Can you work these out from the drawing? Everything is in mm from the part's minimum corner. A direction names the side the tool comes from. Round coordinates to 2 decimals unless told otherwise and drop trailing zeros. Write each loop counter-clockwise with the first axis right and the second up, starting at its lowest first coordinate (ties: lowest second). Pieces come first, ordered by that corner, then holes. Notation, with made-up numbers: M 30,73 L 58,73 A23 cw 58,101 Z; hole C 26,73 d5. An arc over 180 degrees is marked long. Use a Markdown table: item, result. Add a question column.
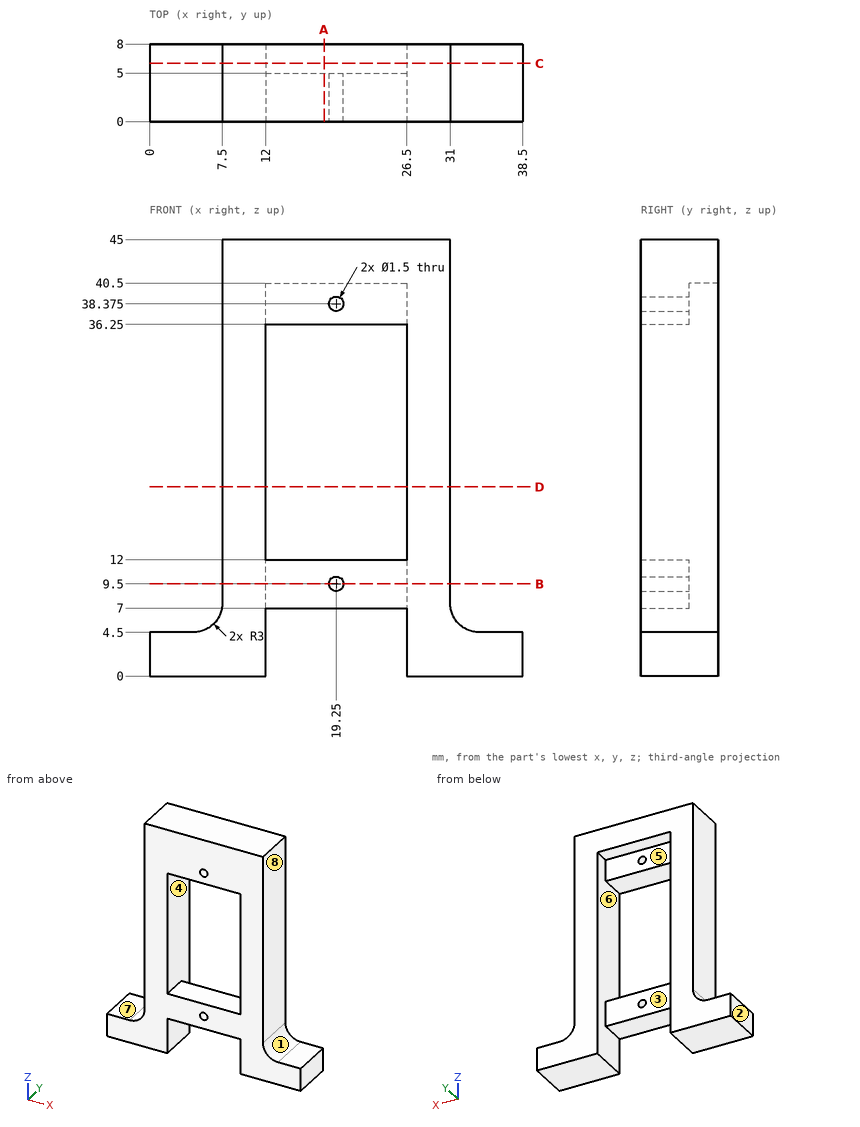
Item 1: Imagine slicing it at C-C on y = 6. List the corners of the cut face in (x, z) for me, plus the area to 3 significant figures.
Item 2: I need wall thicknesses on probe 1 along Z at (x, y) = (19.25, 1.4) (3 decimals); probe 2 along Z at (x, y) = (23.5, 4.5); probe 3 along X at (y, z) = (0.75, 17). Which ranges of each line are inside material? Lowest first, please. Write a range as from..to.
Item 3: Imagine slicing it at A-A on x = 18. List the corners of the cut face in (y, z) for me.
Item 4: For pin 1 Ø3.5 at (x, y) = (1.5, 4.5) entering from +Z; pin 2 Ø1.7 at (x, z) = (19.25, 38.375) entering from +Y; pin 3 Ø0.9 at (x, z) = (19.25, 9.5) entering from +Y; pin 4 Ø2.5 at (x, y) = (17, 6.5) entering from -Z, each with a flat end and sliding along its axis, tell me the tip position at first contact or that it passes through.
Item 5: Imagine slicing it at D-D on z = 19.5. List the corners of the cut face in (x, y) for me.
Item 6: If we mould it in two halves opening along X, with no side actions, what happens to the marked faces 1, 2, 3 and 4? For each: +X half, -X half, draft (parallel to the pull), parting line (faces both ways), or undercut.
Item 7: On a 3-axis mill with a long thin cutter (end or side, diameter ignored), from which of +Z, -Z, +X, -X, +Y, -Y can I reach the whole of each face in a straight line? I mean the marked faces 5, 6, 7 and 8. Say none if no direction works.
Item 8: Imagine slicing it at B-B on z = 9.5. List the corners of the cut face in (x, y) for me.
The answers:
| question | item | result |
|---|---|---|
| 1 | outline | M 0,0 L 12,0 L 12,40.5 L 26.5,40.5 L 26.5,0 L 38.5,0 L 38.5,4.5 L 34,4.5 A3 cw 31,7.5 L 31,45 L 7.5,45 L 7.5,7.5 A3 cw 4.5,4.5 L 0,4.5 Z |
| 1 | area | 542 mm² |
| 2 | probe 1 | 7..8.75, 10.25..12, 36.25..37.625, 39.125..45 |
| 2 | probe 2 | 7..12, 36.25..45 |
| 2 | probe 3 | 7.5..12, 26.5..31 |
| 3 | outline | M 0,7 L 5,7 L 5,12 L 0,12 Z; M 0,36.25 L 5,36.25 L 5,40.5 L 8,40.5 L 8,45 L 0,45 Z |
| 4 | pin 1 | z = 4.5 |
| 4 | pin 2 | y = 5 |
| 4 | pin 3 | through |
| 4 | pin 4 | z = 40.5 |
| 5 | outline | M 7.5,0 L 12,0 L 12,8 L 7.5,8 Z; M 26.5,0 L 31,0 L 31,8 L 26.5,8 Z |
| 6 | face 1 | +X half |
| 6 | face 2 | -X half |
| 6 | face 3 | undercut |
| 6 | face 4 | undercut |
| 7 | face 5 | -Z, +Y |
| 7 | face 6 | +Y |
| 7 | face 7 | +Z, -X, +Y, -Y |
| 7 | face 8 | +Z, +X, +Y, -Y |
| 8 | outline | M 7.5,0 L 18.5,0 L 18.5,5 L 12,5 L 12,8 L 7.5,8 Z; M 20,0 L 31,0 L 31,8 L 26.5,8 L 26.5,5 L 20,5 Z |
